Read the model definition and answer for the solid it produces. Units are mm, in the model's axes. A direction names the side the tool comes from. Give positions to 0.01 mm unless a question says otherwise; leave off trailing zeros. Loops run counter-clockwise (first coordinate to the right, second up) from the corner with the lowest first, then second, coordinate; pieces in that order, holes last. Notation, with made-up numbers: (82, 31.25) -> (133, 31.25) arc R18 cw to (133, 61.25) -> close; hole circle Ø7 at (45.25, 45.25). An arc over 180 degrees is marked (long way). Write each question's results on one line, items separated by ' | '. Start each with the question number.
Item 1: Determine the mould class of faces 3 (the conical face through (-0.146, 4.126, 10.022)), 4 (the cylindrical face through (-5.436, -1.723, 5.147)), 5 (the flat face through (0, 6.655, 5)), 6 (the flat face through (0.635, 6, 5)) for opening direction Y: +Y half, -Y half, draft (parallel to the pull), parting line (faces both ways), or undercut.
Item 2: Which of the six approach directions +Z, -Z, +X, -X, +Y, -Y give full straight-line access (tool end or side, diameter ignored) to faces 1 (the flat face through (5.67, 2.51, 5.15)), 2 (the flat face through (-1, -4, 10.439))?
Item 3: Section B-B on y = 0 is taken. Write down the section's boundary in (x, z), and give its area (3 significant figures).
Item 4: Section D-D on y = -4.5 is taken. Write down the section's boundary in (x, z).
Item 5: Each of these flat-tipped pins is pushed along its axis until it touches: P1, Ø6, axis at x = 5, z = 1.5, coming from the +Y side; P2, Ø0.5, axis at y = 6, z = 3, coming from the -X side (3 decimals); P3, Ø1, axis at x = -5, z = 3.5, coming from the +Y side. Where does it stop, or does it pass through?
Item 6: Section C-C on z = 9.25 is taken. Write down the section's boundary in (x, y) (3 decimals).
Item 7: Section A-A on x = 0 is taken. Write down the section's boundary in (y, z), and give its area (3 significant figures).
Item 8: Find the intervals of material crossed by line 1 (Y direction, x = 0, z = 5); line 2 (X direction, y = 0, z = 7.75); line 3 (X direction, y = 2.25, z = 2.75), in increasing order.
```python
from build123d import *

# Parameters (mm, degrees)
F1_DEPTH = 10.4394
F2_SIZE  = 0.5842


with BuildPart() as f1:
    # F0 (on Top) → F1 (new body)
    with BuildSketch(Plane.XY):
        with BuildLine():
            Line((-6.525317, 1.452525), (-5.585705, 1.147227))
            ThreePointArc((-5.585705, 1.147227), (-5.42321, -1.762108), (-3.844607, -4.211321))
            Line((-3.844607, -4.211321), (-4.425319, -5.010603))
            Line((-4.425319, -5.010603), (-3.397868, -5.75709))
            Line((-3.397868, -5.75709), (-2.817155, -4.957808))
            ThreePointArc((-2.817155, -4.957808), (0, -5.7023), (2.817155, -4.957808))
            Line((2.817155, -4.957808), (3.397868, -5.75709))
            Line((3.397868, -5.75709), (4.425319, -5.010603))
            Line((4.425319, -5.010603), (3.844607, -4.211321))
            ThreePointArc((3.844607, -4.211321), (5.42321, -1.762108), (5.585705, 1.147227))
            Line((5.585705, 1.147227), (6.525317, 1.452525))
            Line((6.525317, 1.452525), (6.132865, 2.660367))
            Line((6.132865, 2.660367), (5.193253, 2.355069))
            ThreePointArc((5.193253, 2.355069), (3.351728, 4.613258), (0.635, 5.666833))
            Line((0.635, 5.666833), (0.635, 6.6548))
            Line((0.635, 6.6548), (-0.635, 6.6548))
            Line((-0.635, 6.6548), (-0.635, 5.666833))
            ThreePointArc((-0.635, 5.666833), (-3.351728, 4.613258), (-5.193253, 2.355069))
            Line((-5.193253, 2.355069), (-6.132865, 2.660367))
            Line((-6.132865, 2.660367), (-6.525317, 1.452525))
        make_face()
        with BuildLine():
            ThreePointArc((-2.404295, -3.1496), (0, 3.9624), (2.404295, -3.1496))
            Line((2.404295, -3.1496), (-2.404295, -3.1496))
        make_face(mode=Mode.SUBTRACT)
    extrude(amount=F1_DEPTH)

    # F2
    f2_edges = [f1.edges().sort_by_distance(p)[0] for p in [
        (0, 3.9624, 10.4394),
        (0, -3.1496, 10.4394),
        (0, -3.1496, 0),
        (0, 3.9624, 0),
    ]]
    chamfer(f2_edges, length=F2_SIZE)


solid = f1.part
```
Findings:
1) face 3: undercut | face 4: undercut | face 5: +Y half | face 6: draft
2) face 1: +Z, -Z, +Y | face 2: +Z, +X, -X, +Y, -Y
3) outline: (-5.7, 0) -> (-4.55, 0) -> (-3.96, 0.58) -> (-3.96, 9.86) -> (-4.55, 10.44) -> (-5.7, 10.44) -> close; (3.96, 0.58) -> (4.55, 0) -> (5.7, 0) -> (5.7, 10.44) -> (4.55, 10.44) -> (3.96, 9.86) -> close | area: 35.6 mm2
4) outline: (-4.05, 0) -> (4.05, 0) -> (4.05, 10.44) -> (-4.05, 10.44) -> close
5) P1: y = 5.34 | P2: x = -0.635 | P3: y = 3.5
6) outline: (-6.525, 1.453) -> (-5.586, 1.147) arc R5.702 ccw to (-3.845, -4.211) -> (-4.425, -5.011) -> (-3.398, -5.757) -> (-2.817, -4.958) arc R5.702 ccw to (2.817, -4.958) -> (3.398, -5.757) -> (4.425, -5.011) -> (3.845, -4.211) arc R5.702 ccw to (5.586, 1.147) -> (6.525, 1.453) -> (6.133, 2.66) -> (5.193, 2.355) arc R5.702 ccw to (0.635, 5.667) -> (0.635, 6.655) -> (-0.635, 6.655) -> (-0.635, 5.667) arc R5.702 ccw to (-5.193, 2.355) -> (-6.133, 2.66) -> close; hole (-2.404, -3.15) -> (2.404, -3.15) arc R3.962 ccw (long way) to start
7) outline: (-5.7, 0) -> (-3.73, 0) -> (-3.15, 0.58) -> (-3.15, 9.86) -> (-3.73, 10.44) -> (-5.7, 10.44) -> close; (3.96, 0.58) -> (4.55, 0) -> (6.65, 0) -> (6.65, 10.44) -> (4.55, 10.44) -> (3.96, 9.86) -> close | area: 54.1 mm2
8) line 1: -5.7 to -3.15, 3.96 to 6.65 | line 2: -5.7 to -3.96, 3.96 to 5.7 | line 3: -6.27 to -3.26, 3.26 to 6.27
